from build123d import *

# Parameters (mm, degrees)
SKETCH1_R           = 2.9
BOSS_EXTRUDE1_DEPTH = 3
SKETCH2_W           = 23.6
SKETCH2_H           = 20.5
BOSS_EXTRUDE2_DEPTH = 3
SKETCH3_W           = 23.6
SKETCH3_H           = 6.2
BOSS_EXTRUDE3_DEPTH = 7
SKETCH4_R           = 2.4
CUT_EXTRUDE2_DEPTH  = 37.390148045
CHAMFER1_SIZE       = 2.8
CHAMFER1_SIZE2      = 1.960581107
CHAMFER2_SIZE       = 1
CHAMFER3_SIZE       = 0.5


with BuildPart() as part:
    # Sketch1 → Boss-Extrude1 (new body)
    with BuildSketch(Plane.XY):
        Polygon((0, 0), (-23.6, 0), (-23.6, -14.4), (-23.6, -18.628818394), (-19.3, -18.628818394), (-4.3, -18.628818394), (0, -18.628818394), (0, -14.256438623), align=None)
        with Locations((-11.8, -12.828818394)):
            Circle(SKETCH1_R, mode=Mode.SUBTRACT)
    extrude(amount=BOSS_EXTRUDE1_DEPTH)

    # Sketch2 → Boss-Extrude2 (add)
    with BuildSketch(Plane(origin=(0, 0, 0), x_dir=(1, 0, 0), z_dir=(0, 1, 0))):
        with Locations((-11.8, 7.25)):
            Rectangle(SKETCH2_W, SKETCH2_H)
    extrude(amount=BOSS_EXTRUDE2_DEPTH)

    # Sketch3 → Boss-Extrude3 (add)
    with BuildSketch(Plane(origin=(0, 3, 0), x_dir=(1, 0, 0), z_dir=(0, 1, 0))):
        with Locations((-11.8, 0.1)):
            Rectangle(SKETCH3_W, SKETCH3_H)
        with Locations((-11.8, 14.4)):
            Rectangle(SKETCH3_W, SKETCH3_H)
    extrude(amount=BOSS_EXTRUDE3_DEPTH)

    # Sketch4 → Cut-Extrude2 (cut, through all)
    with BuildSketch(Plane.XY.offset(3)):
        with Locations((-11.8, 6.5)):
            Circle(SKETCH4_R)
        with Locations((-19.8, 6.5)):
            Circle(SKETCH4_R)
        with Locations((-3.8, 6.5)):
            Circle(SKETCH4_R)
    extrude(amount=-CUT_EXTRUDE2_DEPTH, mode=Mode.SUBTRACT)

    # Chamfer1
    chamfer1_edges = [part.edges().sort_by_distance(p)[0] for p in [
        (-23.6, -18.628818394, 1.5),
        (-23.6, 10, -0.1),
        (-23.6, 10, -14.4),
    ]]
    chamfer1_side = [part.faces().sort_by_distance(p)[0] for p in [
        (-23.6, 0.665571513, -4.855098328),
    ]]
    chamfer(chamfer1_edges, length=CHAMFER1_SIZE, length2=CHAMFER1_SIZE2, reference=chamfer1_side[0])

    # Chamfer2
    chamfer2_edges = [part.edges().sort_by_distance(p)[0] for p in [
        (-14.7, -12.828818394, 3),
    ]]
    chamfer(chamfer2_edges, length=CHAMFER2_SIZE)

    # Chamfer3
    chamfer3_edges = [part.edges().sort_by_distance(p)[0] for p in [
        (-6.2, 6.5, -3.2),
        (-6.2, 6.5, -17.5),
        (-6.2, 6.5, -11.3),
        (-6.2, 6.5, 3),
        (-22.2, 6.5, -3.2),
        (-22.2, 6.5, -17.5),
        (-22.2, 6.5, -11.3),
        (-22.2, 6.5, 3),
        (-14.2, 6.5, -3.2),
        (-14.2, 6.5, -17.5),
        (-14.2, 6.5, -11.3),
        (-14.2, 6.5, 3),
    ]]
    chamfer(chamfer3_edges, length=CHAMFER3_SIZE)


solid = part.part
CAD build for the part. Positions are in the model's coordinates, mm. A direction names the side the tool comes from. Give positions to 0.01 mm unless a question says otherwise; leave off trailing zeros. Order: outer loops, then holes, each group sorted by start corner. A loop starts at its lowest first (then second) coordinate and runs counter-clockwise, first axis right, second up. Notation, with made-up numbers: (46, 6) -> (67, 6) arc R20 ccw to (67, 11) -> close; hole circle Ø11 at (-21.75, 59). An arc over 180 degrees is marked (long way). Return JSON: item names as keys, results as strings.
Q1. Which spindle directions (+Z, -Z, +X, -X, +Y, -Y) get a long thin tool onto all of the face, cutting with end or side? Do faces 5 (the face through (-12, -9, 0)), 6 (the face through (-15, 6, -11.3)), 7 (the face through (-22.606, -17.248, 1.479)). Say none if no direction does.
Working result:
{"face 5": "-Z, +X, -X, -Y", "face 6": "+X, -X, +Y", "face 7": "+Z, -Z, -X, -Y"}
Q2. Saw through at B-B (x = -3.8). Write the cut outline in (y, z), then the cut area to 3 significant figures.
Working result:
{"outline": "(-18.63, 0) -> (0, 0) -> (0, -17.5) -> (3.6, -17.5) -> (4.1, -17) -> (4.1, -11.8) -> (3.6, -11.3) -> (3, -11.3) -> (3, -3.2) -> (3.6, -3.2) -> (4.1, -2.7) -> (4.1, 2.5) -> (3.6, 3) -> (-18.63, 3) -> close; (8.9, -17) -> (9.4, -17.5) -> (10, -17.5) -> (10, -11.3) -> (9.4, -11.3) -> (8.9, -11.8) -> close; (8.9, -2.7) -> (9.4, -3.2) -> (10, -3.2) -> (10, 3) -> (9.4, 3) -> (8.9, 2.5) -> close", "area": "144 mm²"}
Q3. Drill centre lines: line 1 (Y direction, x = -3.8, z = -15.1); line 2 (Y direction, x = -11.8, z = 1.2); line 3 (Z direction, x = -1.25, y = -11.5). Where is each one in solid material? Low to high.
Working result:
{"line 1": "0 to 4.1, 8.9 to 10", "line 2": "-18.63 to -15.73, -9.93 to 4.1, 8.9 to 10", "line 3": "0 to 3"}
Q4. Mould opens along Y. For faces 1 (the face through (-9.583, 5.581, -0.064)), 2 (the face through (-6.198, 6.606, -0.064)), 3 (the face through (0, 1, -5)), 4 (the face through (-12, 0, -9)) say: pulls with the +Y half, pulls with the -Y half, needs draft (parallel to the pull), parting line crosses it, or undercut.
Working result:
{"face 1": "undercut", "face 2": "undercut", "face 3": "needs draft", "face 4": "pulls with the -Y half"}
Q5. Saw through at A-A (z = -15). Write the cut outline in (x, y).
Working result:
{"outline": "(-23.6, 0) -> (0, 0) -> (0, 10) -> (-21.64, 10) -> (-23.6, 7.2) -> close; hole circle Ø4.8 at (-19.8, 6.5); hole circle Ø4.8 at (-11.8, 6.5); hole circle Ø4.8 at (-3.8, 6.5)"}
Q6. Flat gauge pins, fed straight in: pin 1 (4 mm diameter, centred on y = -11, z = -3, fed in from +X); pin 2 (1.5 mm diameter, centred on x = -17, z = -9.5, fed in from +Y); pin 3 (4 mm diameter, centred on x = -12.5, z = -13.5, fed in from -Y); pin 4 (5.5 mm diameter, centred on x = -19.8, y = 6.5, fed in from -Z). Where does each tip first touch, or does it go through?
Working result:
{"pin 1": "through", "pin 2": "y = 3", "pin 3": "y = 0", "pin 4": "z = -17.35"}
Q7. Saw through at C-C (x = -11.8). Count the separate pieces of the cut face and the enclosed holes in it, then the cut area to 3 significant figures.
Working result:
{"separate pieces": "4", "enclosed holes": "0", "area": "125 mm²"}
